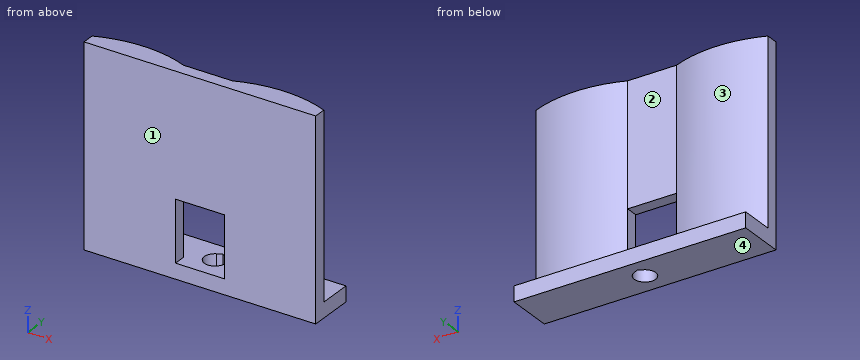
from build123d import *

# Parameters (mm, degrees)
SKETCH1_W           = 38
SKETCH1_H           = 7.5
BOSS_EXTRUDE1_DEPTH = 2.5
BOSS_EXTRUDE5_DEPTH = 30
SKETCH7_W           = 8
SKETCH7_H           = 2
BOSS_EXTRUDE6_DEPTH = 20


with BuildPart() as part:
    # Sketch1 → Boss-Extrude1 (new body)
    with BuildSketch(Plane.XY):
        Rectangle(SKETCH1_W, SKETCH1_H)
        with BuildLine():
            Line((0, 1.961391495), (0.790288933, 1.561391495))
            ThreePointArc((0.790288933, 1.561391495), (0, -1.75), (-0.790288933, 1.561391495))
            Line((-0.790288933, 1.561391495), (0, 1.961391495))
        make_face(mode=Mode.SUBTRACT)
    extrude(amount=BOSS_EXTRUDE1_DEPTH)

    # Sketch6 → Boss-Extrude5 (add)
    with BuildSketch(Plane.XY.offset(2.5)):
        with BuildLine():
            Line((-19, -3.75), (-19, -1.75))
            ThreePointArc((-19, -1.75), (-11.5, -0.290496218), (-4, -1.75))
            Line((-4, -1.75), (-4, -3.75))
            Line((-4, -3.75), (-19, -3.75))
        make_face()
    boss_extrude5 = extrude(amount=BOSS_EXTRUDE5_DEPTH)

    # Mirror1: Boss-Extrude5 across plane
    add(boss_extrude5.mirror(Plane(origin=(0, 0, 0), x_dir=(0, 0, 1), z_dir=(1, 0, 0))))

    # Sketch7 → Boss-Extrude6 (add)
    with BuildSketch(Plane.XY.offset(32.5)):
        with Locations((0, -2.75)):
            Rectangle(SKETCH7_W, SKETCH7_H)
    extrude(amount=-BOSS_EXTRUDE6_DEPTH)


solid = part.part
Can you work these out from the model? Positions are in its coordinate system, mm. Face numbers are marked on the shaded views. A direction names the side the tool comes from. Give positions to 0.01 mm unless a question says otherwise; leave off trailing zeros. Order: outer loops, then holes, each group sorted by start corner. A loop starts at its lowest first (then second) coordinate and runs counter-clockwise, first axis right, second up. Notation, with made-up numbers: M 7,-28.75 L 41,-28.75 A27 cw 41,-5.75 Z; hole C 46.5,45.5 d7. An arc over 180 degrees is marked long. One line per question, with ' | ' between items.
Item 1: We'd pull the mould along X, two halves only. Please class the marked faces 3 and 4: released by +X, released by -X, zero draft, split by the parting line, or undercut.
Answer block:
face 3: undercut | face 4: zero draft
Item 2: Suppose I cut it at C-C, the plane z = 13. Write out the boundary of the cut face in (x, y), then the cut area to 3 significant figures.
Answer block:
outline: M -19,-3.75 L 19,-3.75 L 19,-1.75 A20 ccw 4,-1.75 L -4,-1.75 A20 ccw -19,-1.75 Z | area: 105 mm2
Item 3: Suppose I cut it at B-B, the plane y = -0.75. Write out the boundary of the cut face in (x, z), then the cut area to 3 significant figures.
Answer block:
outline: M -19,0 L -1.58,0 L -1.58,2.5 L -7.24,2.5 L -7.24,32.5 L -15.76,32.5 L -15.76,2.5 L -19,2.5 Z; M 1.58,0 L 19,0 L 19,2.5 L 15.76,2.5 L 15.76,32.5 L 7.24,32.5 L 7.24,2.5 L 1.58,2.5 Z | area: 599 mm2
Item 4: Please list where these lines run through material, in increasing order: L1, parallel to X at y = -2, z = 9; L2, parallel to X at y = 0, z = 1.8; L3, parallel to Y at x = 0, z = 1.9.
Answer block:
L1: x = -19 to -4, 4 to 19 | L2: x = -19 to -1.75, 1.75 to 19 | L3: y = -3.75 to -1.75, 1.96 to 3.75
Item 5: I'm going to push flat-ended pins straight in: pin 1 Ø12 at (x, z) = (14.5, 25.5) entering from +Y; pin 2 Ø3 at (x, z) = (-1.5, 28.5) entering from +Y; pin 3 Ø6 at (x, z) = (-1.5, 18) entering from +Y. Where does each tip first touch, or does it pass through?
Answer block:
pin 1: stops at y = -0.29 | pin 2: stops at y = -1.75 | pin 3: stops at y = -1.56
Item 6: Suppose I cut it at D-D, the plane x = 11.5. Write out the boundary of the cut face in (y, z).
Answer block:
outline: M -3.75,0 L 3.75,0 L 3.75,2.5 L -0.29,2.5 L -0.29,32.5 L -3.75,32.5 Z
Item 7: Suppose I cut it at A-A, the plane x = 3.5. Write out the boundary of the cut face in (y, z).
Answer block:
outline: M -3.75,0 L 3.75,0 L 3.75,2.5 L -3.75,2.5 Z; M -3.75,12.5 L -1.75,12.5 L -1.75,32.5 L -3.75,32.5 Z
Item 8: For the marked faces 1 and 2, which set-ups out of +Z, -Z, +X, -X, +Y, -Y let a thin tool reach every point of the face, with its end or its side?
Answer block:
face 1: +Z, -Z, +X, -X, -Y | face 2: +Z, +Y
